Geometry: final body of the model. Coordinates: model frame, mm. Face numbers are marked on the shaded views. A direction names the side the tool comes from. Give positions to 0.01 mm unless a question says otherwise; leave off trailing zeros. Order: outer loops, then holes, each group sorted by start corner. A loop starts at its lowest first (then second) coordinate and runs counter-clockwise, first axis right, second up. Notation, with made-up numbers: M -37,67 L -19,67 A27 ccw -19,98 Z; hole C 12.25,-40 d10. An arc over 180 degrees is marked long. One line per item, written item: value. Start each with the question number.
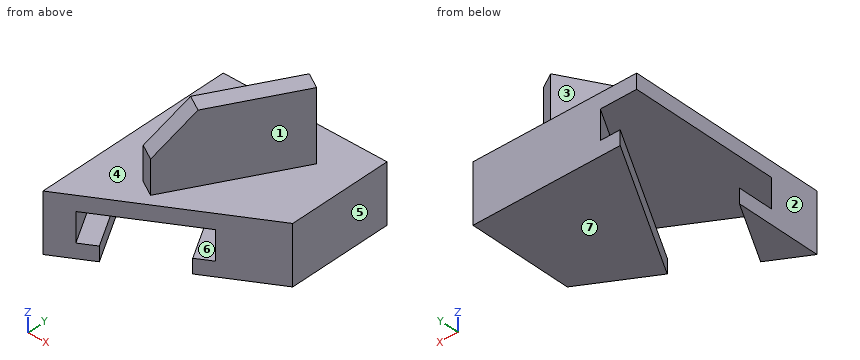
```python
from build123d import *

# Parameters (mm, degrees)
F1_DEPTH = 31.75
F3_DEPTH = 120
F5_DEPTH = 38.1
F6_SIZE  = 20


with BuildPart() as f1:
    # F0 (on Top) → F1 (new body)
    with BuildSketch(Plane.XY):
        Polygon((88.9, 107.55), (0, 107.55), (0, 0), (88.9, 51.326438931), align=None)
    extrude(amount=F1_DEPTH)

    # F2 (on face) → F3 (cut)
    with BuildSketch(Plane(origin=(0, 0, 0), x_dir=(0.8660254038, 0.5, 0), z_dir=(0.5, -0.8660254038, 0))):
        Polygon((70.9, 23.62), (13.5, 23.62), (13.5, 7.87), (23.15, 7.87), (23.15, 0), (61.55, 0), (61.55, 7.87), (70.9, 7.87), align=None)
    extrude(amount=-F3_DEPTH, mode=Mode.SUBTRACT)

    # F4 (on face) → F5 (join)
    with BuildSketch(Plane.XY.offset(31.75)):
        Polygon((33.9, 26.9282217351), (68.9, 87.55), (60.4562523131, 92.425), (25.4562523131, 31.8032217351), align=None)
    extrude(amount=F5_DEPTH)

    # F6
    f6_edges = [f1.edges().sort_by_distance(p)[0] for p in [
        (29.678126, 29.365722, 69.85),
    ]]
    chamfer(f6_edges, length=F6_SIZE)


solid = f1.part
```
Q1. Section query C-C on y = 80. Return loops of the section in (x, z).
Q2. Contact query for flat-ended pins moving along their axis: pin 1 (5 mm diameter, centred on y = 84.5, z = 54.5, fed in from -X); pin 2 (10 mm diameter, centred on x = 14, y = 26, fed in from +Z); pin 3 (5 mm diameter, centred on x = 32, z = 58.5, fed in from -Y); pin 4 (1 mm diameter, centred on y = 88.5, z = 27.5, fed in from -X). Output: stop coordinate, or through.
Q3. Set-up query: the marked faces 1, 2 and 3. Return all of +Z, -Z, +X, -X, +Y, -Y with unobstructed straight access to the full face (end or side cutting, diameter ignored); none if empty.
Q4. Ray query, line 1 along Z through (x, y) = (9.5, 25); line 2 along Z through (x, y) = (27.5, 52.5); line 3 along Z through (x, y) = (83.5, 55). Return the intervals inside material, ascending. Write a range as [from, to].
Q5. Mould query, pull axis Z, two halves, no side actions, for the marked faces 4, 5, 6 and 7. Classes: +Z half, -Z half, draft (parallel to the pull), parting line (faces both ways), or undercut.
Q6. Section query D-D on x = 66. Return loops of the section in (y, z), and give its area (3 significant figures).
Q7. Section query A-A on z = 5. Return loops of the section in (x, y) (3 decimals).
Q8. Section query B-B on z = 19.5. Return loops of the section in (x, y), and give its area (3 significant figures).
Results below:
1. outline: M 0,23.62 L 35.68,23.62 L 35.68,7.87 L 24.88,7.87 L 24.88,0 L 88.9,0 L 88.9,31.75 L 64.54,31.75 L 64.54,69.85 L 53.28,69.85 L 53.28,31.75 L 0,31.75 Z
2. pin 1: x = 54.44
2. pin 2: z = 31.75
2. pin 3: y = 34.79
2. pin 4: x = 0
3. face 1: +Z, +X, -Y
3. face 2: +Z, -Z, -X, +Y, -Y
3. face 3: +Z, -X, +Y
4. line 1: [0, 7.87], [23.62, 31.75]
4. line 2: [23.62, 31.75]
4. line 3: [0, 31.75]
5. face 4: +Z half
5. face 5: draft
5. face 6: undercut
5. face 7: -Z half
6. outline: M 38.11,0 L 107.55,0 L 107.55,31.75 L 89.22,31.75 L 89.22,69.85 L 82.53,69.85 L 82.53,31.75 L 38.11,31.75 Z
6. area: 2,460 mm2
7. outline: M 0,0 L 20.048,11.575 L 0,46.3 Z; M 8.978,107.55 L 53.304,30.775 L 88.9,51.326 L 88.9,107.55 Z
8. outline: M 0,0 L 11.69,6.75 L 0,27 Z; M 19.77,107.55 L 61.4,35.45 L 88.9,51.33 L 88.9,107.55 Z
8. area: 3,420 mm2
